from build123d import *

# Parameters (mm, degrees)
SKETCH2_W           = 2.5
SKETCH2_H           = 2.5
BOSS_EXTRUDE1_DEPTH = 7.05
PINHOLE_REACH       = 16.1
SKETCH3_W           = 0.67
SKETCH3_H           = 0.63
CUT_EXTRUDE2_DEPTH  = 0.35
SKETCH5_W           = 2.1
SKETCH5_H           = 5.3
CUT_EXTRUDE3_DEPTH  = 1.215
CUT_EXTRUDE5_DEPTH  = 0.025
SKETCH7_W           = 2.1
SKETCH7_H           = 2.1
CUT_EXTRUDE6_DEPTH  = 4
SKETCH9_W           = 0.15
SKETCH9_H           = 1
HOLDER_1_DEPTH      = 1.065
SKETCH10_W          = 1.8
SKETCH10_H          = 1
HOLDER_2_DEPTH      = 0.15


with BuildPart() as part:
    # Sketch2 → Boss-Extrude1 (new body, symmetric)
    with BuildSketch(Plane(origin=(0, 0, 0), x_dir=(1, 0, 0), z_dir=(0, 1, 0))):
        Rectangle(SKETCH2_W, SKETCH2_H)
    extrude(amount=BOSS_EXTRUDE1_DEPTH, both=True)

    # Sketch3 → Pinhole (cut, up to next)
    with BuildSketch(Plane(origin=(0, 7.05, 0), x_dir=(1, 0, 0), z_dir=(0, 1, 0)), mode=Mode.PRIVATE) as pinhole_sk1:
        Rectangle(SKETCH3_W, SKETCH3_H)
    pinhole_tool1 = extrude(pinhole_sk1.sketch, amount=-PINHOLE_REACH, mode=Mode.PRIVATE) & part.part
    add(pinhole_tool1.solids().sort_by_distance((0, 7.05, 0))[0], mode=Mode.SUBTRACT)

    # Sketch4 → Cut-Extrude2 (cut)
    with BuildSketch(Plane.XY.offset(1.25)):
        Polygon((-1.25, 3.25), (1.25, 3.25), (1.25, -2.05), (0.675, -2.05), (0.675, 1.55), (-0.675, 1.55), (-0.675, -2.05), (-1.25, -2.05), align=None)
    extrude(amount=-CUT_EXTRUDE2_DEPTH, mode=Mode.SUBTRACT)

    # Sketch5 → Cut-Extrude3 (cut)
    with BuildSketch(Plane.XY.offset(0.9)):
        with Locations((0, 0.6)):
            Rectangle(SKETCH5_W, SKETCH5_H)
    extrude(amount=-CUT_EXTRUDE3_DEPTH, mode=Mode.SUBTRACT)

    # Sketch6 → Cut-Extrude5 (cut)
    with BuildSketch(Plane.XY.offset(1.25)):
        with BuildLine():
            Line((-0.575, 0.825), (-0.575, -2.05))
            Line((-0.575, -2.05), (0.575, -2.05))
            Line((0.575, -2.05), (0.575, 0.825))
            ThreePointArc((0.575, 0.825), (0, 1.4), (-0.575, 0.825))
        make_face()
    extrude(amount=-CUT_EXTRUDE5_DEPTH, mode=Mode.SUBTRACT)

    # Sketch7 → Cut-Extrude6 (cut)
    with BuildSketch(Plane.XZ.offset(7.05)):
        Rectangle(SKETCH7_W, SKETCH7_H)
    extrude(amount=-CUT_EXTRUDE6_DEPTH, mode=Mode.SUBTRACT)

    # Sketch9 → Holder-1 (add)
    with BuildSketch(Plane.XY.offset(-0.315)):
        with Locations((-0.825, 2.4)):
            Rectangle(SKETCH9_W, SKETCH9_H)
        with Locations((0.825, 2.4)):
            Rectangle(SKETCH9_W, SKETCH9_H)
    extrude(amount=HOLDER_1_DEPTH)

    # Sketch10 → Holder-2 (add)
    with BuildSketch(Plane.XY.offset(0.75)):
        with Locations((0, 2.4)):
            Rectangle(SKETCH10_W, SKETCH10_H)
    extrude(amount=HOLDER_2_DEPTH)


solid = part.part
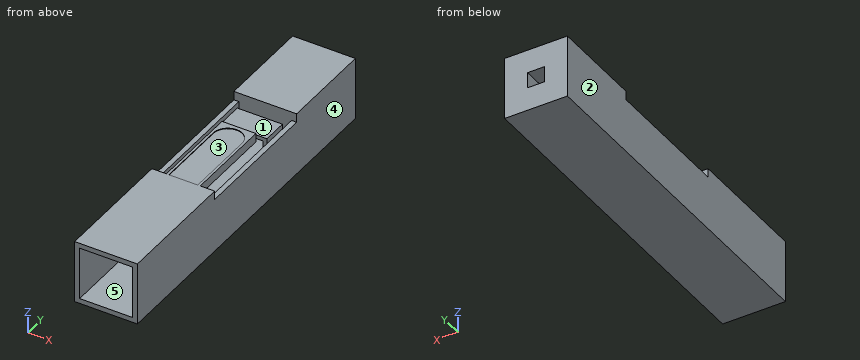
Model file for the job. Use its own axes, mm. Face numbers are marked on the shaded views. A direction names the side the tool comes from. Give positions to 0.01 mm unless a question says otherwise; leave off trailing zeros. Loops run counter-clockwise (first coordinate to the right, second up) from the corner with the lowest first, then second, coordinate; pieces in that order, holes last. Notation, with made-up numbers: (-5, 38.5) -> (10, 38.5) arc R21 ccw to (10, 60.5) -> close; hole circle Ø6 at (31.5, -24). An arc over 180 degrees is marked (long way). Use a Markdown table: item, result. Add a question column.
(1) Slice it at B-B on z = 0.1. List the corners of the cut face in (x, y) (3 decimals).
(2) Slice it at A-A on y = 3.75. List the corners of the cut face in (x, z) (3 decimals), and give its area (3 significant figures).
(3) Drop a flat-ended pin along its axis: pin 1 Ø1 at (x, z) = (-0.5, 0.5) entering from -Y. Give the stop position or say it passes through.
(4) Slice it at C-C on x = 0. List the corners of the cut face in (y, z) (3 decimals), and give its area (3 significant figures).
(5) Wall check: line 1 along X through (y, z) = (2.75, 0.6); line 2 along Z through (x, y) = (-0.2, 5.75) (3 decimals); line 3 along Y through (x, z) = (0.5, 1). Give the ranges that are in metal, low to high.
(6) Slice it at D-D on z = -0.55. List the corners of the cut face in (x, y), and give its area (4 significant figures).
(7) Mould opens along X. For the marked faces 1, 2 and 3 say: +X half, -X half, draft (parallel to the pull), parting line (faces both ways), or undercut.
(8) Tool access for the marked faces 4 and 5: list every direction of +Z, -Z, +X, -X, +Y, -Y with a clear straight run to the whole face (end or side of a thin tool).
Filled sheet:
| question | item | result |
|---|---|---|
| 1 | outline | (-1.25, -7.05) -> (-1.05, -7.05) -> (-1.05, -3.05) -> (-0.335, -3.05) -> (-0.335, -2.05) -> (-1.05, -2.05) -> (-1.05, 3.25) -> (-0.335, 3.25) -> (-0.335, 7.05) -> (-1.25, 7.05) -> close; (-0.9, 1.9) -> (-0.75, 1.9) -> (-0.75, 2.9) -> (-0.9, 2.9) -> close; (0.335, -3.05) -> (1.05, -3.05) -> (1.05, -7.05) -> (1.25, -7.05) -> (1.25, 7.05) -> (0.335, 7.05) -> (0.335, 3.25) -> (1.05, 3.25) -> (1.05, -2.05) -> (0.335, -2.05) -> close; (0.75, 1.9) -> (0.9, 1.9) -> (0.9, 2.9) -> (0.75, 2.9) -> close |
| 2 | outline | (-1.25, -1.25) -> (1.25, -1.25) -> (1.25, 1.25) -> (-1.25, 1.25) -> close; hole (-0.335, -0.315) -> (0.335, -0.315) -> (0.335, 0.315) -> (-0.335, 0.315) -> close |
| 2 | area | 5.83 mm2 |
| 3 | pin 1 | y = -3.05 |
| 4 | outline | (-7.05, -1.25) -> (7.05, -1.25) -> (7.05, -0.315) -> (-3.05, -0.315) -> (-3.05, -1.05) -> (-7.05, -1.05) -> close; (-7.05, 1.05) -> (-3.05, 1.05) -> (-3.05, 0.315) -> (-2.05, 0.315) -> (-2.05, 0.9) -> (1.55, 0.9) -> (1.55, 1.25) -> (1.4, 1.25) -> (1.4, 1.225) -> (-2.05, 1.225) -> (-2.05, 1.25) -> (-7.05, 1.25) -> close; (1.9, 0.75) -> (2.9, 0.75) -> (2.9, 0.9) -> (1.9, 0.9) -> close; (3.25, 0.315) -> (7.05, 0.315) -> (7.05, 1.25) -> (3.25, 1.25) -> close |
| 4 | area | 16.9 mm2 |
| 5 | line 1 | -1.25 to -1.05, -0.9 to -0.75, 0.75 to 0.9, 1.05 to 1.25 |
| 5 | line 2 | -1.25 to -0.315, 0.315 to 1.25 |
| 5 | line 3 | -3.05 to 1.55, 3.25 to 7.05 |
| 6 | outline | (-1.25, -7.05) -> (-1.05, -7.05) -> (-1.05, -3.05) -> (1.05, -3.05) -> (1.05, -7.05) -> (1.25, -7.05) -> (1.25, 7.05) -> (-1.25, 7.05) -> close |
| 6 | area | 26.85 mm2 |
| 7 | face 1 | draft |
| 7 | face 2 | -X half |
| 7 | face 3 | undercut |
| 8 | face 4 | +Z, -Z, +X, +Y, -Y |
| 8 | face 5 | -Y |
